Here's how the part is built. I have some questions about the finished solid (model axes, mm). A direction names the side the tool comes from. Coordinates: 2 decimals unless noted, no trailing zeros. Order: outer loops, then holes, each group sorted by start corner. A loop starts at its lowest first (then second) coordinate and runs counter-clockwise, first axis right, second up. Notation, with made-up numbers: (-9, 62.5) - (3, 62.5) arc R27 ccw to (3, 88.5) - close; hole circle Ø11 at (-16, -13.5). An arc over 180 degrees is marked (long way). Use one line per item in the form item = value. Start each with the question number.
from build123d import *

# Parameters (mm, degrees)
F0_W     = 50
F0_H     = 50
F0_W_2   = 40
F0_H_2   = 40
F1_DEPTH = 50
F2_W     = 40
F2_H     = 5
F3_DEPTH = 40


with BuildPart() as f1:
    # F0 (on Top) → F1 (new body)
    with BuildSketch(Plane.XY):
        Rectangle(F0_W, F0_H)
        Rectangle(F0_W_2, F0_H_2, mode=Mode.SUBTRACT)
    extrude(amount=F1_DEPTH)

    # F2 (on face) → F3 (join)
    with BuildSketch(Plane.XZ.offset(-20)):
        with Locations((0, 2.5)):
            Rectangle(F2_W, F2_H)
    extrude(amount=F3_DEPTH)


solid = f1.part
1) For pin 1 (12 mm diameter, centred on x = 8.5, y = -1, fed in from +Z), with a flat end and sliding along its axis, tell me the tip position at first contact or that it passes through.
2) Which directions (+Z, -Z, +X, -X, +Y, -Y) give clear straight access to the entire face, cutting with the end or side of a thin tool? Please do faces 5 (the flat face through (25, 0, 25)), 6 (the flat face through (0, -20, 27)).
3) Suppose I cut it at A-A, the plane z = 28. List the corners of the cut face in (x, y) for me, then the cut area to 3 significant figures.
4) If we mould it in two halves opening along Y, with no side actions, what happens to faces 1 (the flat face through (0, 25, 25)), 2 (the flat face through (0, 0, 5)), 3 (the flat face through (0, -25, 25)), 4 (the flat face through (-25, 0, 25))? For each: pulls with the +Y half, pulls with the -Y half, needs draft (parallel to the pull), parting line crosses it, or undercut.
5) I need wall thicknesses on probe 1 along Y at (x, z) = (-12, 25.5); probe 2 along Z at (x, y) = (-1, -18.5). Which ranges of each line are inside material? Lowest first, please. Write a range as [from, to].
6) Suppose I cut it at B-B, the plane x = 2. List the corners of the cut face in (y, z) for me, then the cut area to 3 significant figures.
From the geometry:
q1.pin_1 = 5
q2.face_5 = +Z, -Z, +X, +Y, -Y
q2.face_6 = +Z
q3.outline = (-25, -25) - (25, -25) - (25, 25) - (-25, 25) - close; hole (-20, -20) - (20, -20) - (20, 20) - (-20, 20) - close
q3.area = 900 mm2
q4.face_1 = pulls with the +Y half
q4.face_2 = undercut
q4.face_3 = pulls with the -Y half
q4.face_4 = needs draft
q5.probe_1 = [-25, -20], [20, 25]
q5.probe_2 = [0, 5]
q6.outline = (-25, 0) - (25, 0) - (25, 50) - (20, 50) - (20, 5) - (-20, 5) - (-20, 50) - (-25, 50) - close
q6.area = 700 mm2
